```python
from build123d import *

# Parameters (mm, degrees)
SKETCH1_W           = 20
SKETCH1_H           = 15
BOSS_EXTRUDE1_DEPTH = 12
SKETCH2_R           = 4
CUT_EXTRUDE1_DEPTH  = 13
CHAMFER1_SIZE       = 2


with BuildPart() as part:
    # Sketch1 → Boss-Extrude1 (new body)
    with BuildSketch(Plane.XY):
        Rectangle(SKETCH1_W, SKETCH1_H)
    extrude(amount=BOSS_EXTRUDE1_DEPTH)

    # Sketch2 → Cut-Extrude1 (cut, through all)
    with BuildSketch(Plane.XY.offset(12)):
        Circle(SKETCH2_R)
    extrude(amount=-CUT_EXTRUDE1_DEPTH, mode=Mode.SUBTRACT)

    # Chamfer1
    chamfer1_edges = [part.edges().sort_by_distance(p)[0] for p in [
        (10, 7.5, 6),
        (10, -7.5, 6),
        (-10, -7.5, 6),
        (-10, 7.5, 6),
    ]]
    chamfer(chamfer1_edges, length=CHAMFER1_SIZE)


solid = part.part
```
The listing builds one solid part. Answer for the finished solid, in the listing's coordinates (mm). Round coordinates to 2 decimals unless told otherwise and drop trailing zeros. Order: outer loops, then holes, each group sorted by start corner. A loop starts at its lowest first (then second) coordinate and runs counter-clockwise, first axis right, second up. Notation, with made-up numbers: (39.25, 11.25) - (63.25, 11.25) arc R18 ccw to (63.25, 22.25) - close; hole circle Ø8 at (9.25, 73). An arc over 180 degrees is marked (long way). Put each result on its own line as item: value. Start each with the question number.
(1) Find section A-A (x = 0). Give the vertices of the cut face in (y, z), plus the area to 3 significant figures.
(2) Find section B-B (y = 0). Give the vertices of the cut face in (x, z), plus the area to 3 significant figures.
(3) Straight lines are drawn through the part: probe 1 along Y at (x, z) = (0, 5); probe 2 along X at (y, z) = (1, 9); probe 3 along X at (y, z) = (-3.5, 3). For each, find the intervals that lie inside material, in ascending order. Write a range as from..to.
(4) Find section D-D (x = 8.5). Give the vertices of the cut face in (y, z), plus the area to 3 significant figures.
(5) Find section C-C (z = 9). Give the vertices of the cut face in (x, y).
(6) Determine the mould class of faces 1 (the flat face through (-9, -6.5, 5.9)), 2 (the cylindrical face through (-0.867, -3.905, 6.084)), 3 (the flat face through (-10, 0, 6)), 4 (the flat face through (0, 7.5, 6)) for opening direction Y: released by +Y, released by -Y, zero draft, split by the parting line, or undercut.
Reply:
1. outline: (-7.5, 0) - (-4, 0) - (-4, 12) - (-7.5, 12) - close; (4, 0) - (7.5, 0) - (7.5, 12) - (4, 12) - close
1. area: 84.0 mm^2
2. outline: (-10, 0) - (-4, 0) - (-4, 12) - (-10, 12) - close; (4, 0) - (10, 0) - (10, 12) - (4, 12) - close
2. area: 144 mm^2
3. probe 1: -7.5..-4, 4..7.5
3. probe 2: -10..-3.87, 3.87..10
3. probe 3: -10..-1.94, 1.94..10
4. outline: (-7, 0) - (7, 0) - (7, 12) - (-7, 12) - close
4. area: 168 mm^2
5. outline: (-10, -5.5) - (-8, -7.5) - (8, -7.5) - (10, -5.5) - (10, 5.5) - (8, 7.5) - (-8, 7.5) - (-10, 5.5) - close; hole circle Ø8 at (0, 0)
6. face 1: released by -Y
6. face 2: undercut
6. face 3: zero draft
6. face 4: released by +Y
